Autodesk Inventor part; units mm, degrees
ref_plane "YZ Plane" through (0, 0, 0) normal (1, 0, 0) x (0, 1, 0)
ref_plane "XZ Plane" through (0, 0, 0) normal (0, 1, 0) x (-1, 0, 0)
ref_plane "XY Plane" through (0, 0, 0) normal (0, 0, 1) x (1, 0, 0)
sketch "Sketch1" plane through (0, 0, 0) normal (0, 0, 1) x (1, 0, 0)
  circle A0 centre (0, 0) radius 6
  line L0 (-5, 0) -> (5, 0)
  line L1 (5, 0) -> (5, -7)
  line L2 (5, -7) -> (-5, -7)
  line L3 (-5, -7) -> (-5, 0)
  point P0 (5, -3.3166)
  point P1 (-5, -3.3166)
  dimension "d0" = 12
  dimension "d1" = 1
  dimension "d2" = 5
  dimension "d3" = 5
extrude "Extrusion1" add sketch "Sketch1" along normal blind 6 contours A0 L1 L2 L3
sketch "Sketch2" plane through (-5, -7, 0) normal (0, -1, 0) x (1, 0, 0)
  line L0 (0, 0) -> (10, 0)
  line L1 (10, 0) -> (10, 6)
  line L2 (0, 6) -> (10, 6)
  line L3 (0, 0) -> (0, 6)
  line L4 (0, 6) -> (10, 6) construction
  line L5 (10, 0) -> (0, 6) construction
  line L6 (0, 0) -> (10, 0) construction
  line L7 (10, 6) -> (0, 0) construction
  circle A0 centre (5, 3) radius 1.55
  point P0 (5, 0)
  dimension "d6" = 3.1
extrude "Extrusion2" cut sketch "Sketch2" along normal mid plane 6 contours A0
properties part number "Tube_adaptor_2"
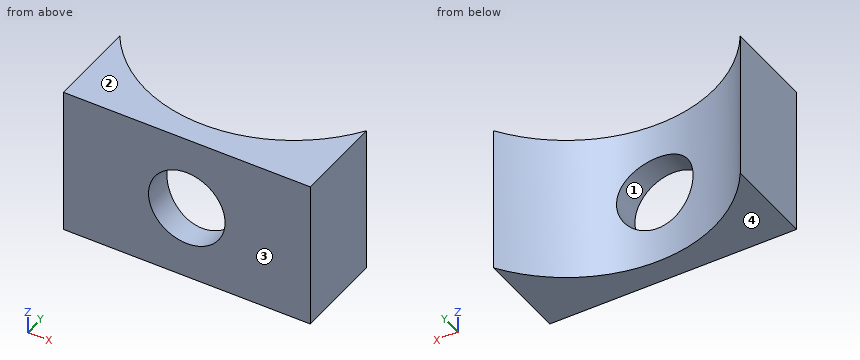
Geometry: final body of the model. Coordinates: model frame, mm. Face numbers are marked on the shaded views. Coordinates: 2 decimals unless noted, no trailing zeros. Loops run counter-clockwise (first coordinate to the right, second up) from the corner with the lowest first, then second, coordinate; pieces in that order, holes last. Notation, with made-up numbers: (8, 38.25) - (13, 38.25) arc R10 cw to (13, 49.25) - close; hole circle Ø4 at (47, 26). An arc over 180 degrees is marked (long way). Put each result on its own line as item: value. Start each with the question number.
Q1. Cut plane A-A, the plane z = 3. Return loops of the section in (x, y), and give its area (3 significant figures).
Q2. Line query: line 1 (Z direction, x = 0, y = -6.65); line 2 (X direction, y = -6.2, z = 3); line 3 (X direction, y = -4.5, z = 4.75). Output: solid intervals per line, ascending.
Q3. Cut plane B-B, the plane x = 0. Return loops of the section in (y, z), and give its area (3 significant figures).
Q4. Cut plane C-C, the plane y = -6.25. Return loops of the section in (x, z).
Q5. Pull-direction query (Z, two-part tool) for the marked faces 1, 2, 3 and 4; classes: released by +Z, released by -Z, zero draft, split by the parting line, or undercut.
Q6. Cut plane D-D, the plane z = 0.75. Return loops of the section in (x, y).
Filled sheet:
1. outline: (-5, -7) - (-1.55, -7) - (-1.55, -5.8) arc R6 cw to (-5, -3.32) - close; (1.55, -7) - (5, -7) - (5, -3.32) arc R6 cw to (1.55, -5.8) - close
1. area: 14.6 mm²
2. line 1: 0 to 1.45, 4.55 to 6
2. line 2: -5 to -1.55, 1.55 to 5
2. line 3: -5 to -3.97, 3.97 to 5
3. outline: (-7, 0) - (-6, 0) - (-6, 1.45) - (-7, 1.45) - close; (-7, 4.55) - (-6, 4.55) - (-6, 6) - (-7, 6) - close
3. area: 2.90 mm²
4. outline: (-5, 0) - (5, 0) - (5, 6) - (-5, 6) - close; hole circle Ø3.1 at (0, 3)
5. face 1: undercut
5. face 2: released by +Z
5. face 3: zero draft
5. face 4: released by -Z
6. outline: (-5, -7) - (5, -7) - (5, -3.32) arc R6 cw to (-5, -3.32) - close
